Design review of the part built by this model. Coordinates are the model's own, in mm. A direction names the side the tool comes from. Give positions to 0.01 mm unless a question says otherwise; leave off trailing zeros. Order: outer loops, then holes, each group sorted by start corner. A loop starts at its lowest first (then second) coordinate and runs counter-clockwise, first axis right, second up. Notation, with made-up numbers: (24, 59) -> (30, 59) arc R21 ccw to (30, 76) -> close; hole circle Ø8 at (28, 74.5). An arc over 180 degrees is marked (long way). One line per item, written item: value. Start each with the question number.
1) Consider section C-C (z = -2.75). State how many separate pieces and enclosed holes the cut face has, plus the area to 3 significant figures.
2) Wall thickness on line 1 along Y through (x, z) = (30, 3.25); line 2 along Y through (x, z) = (70, -2.5); line 3 along Y through (x, z) = (11.5, 4.5): over which ranges is each line inside the solid? List them lowest first. Write a range as from..to.
3) Tool access review of faces 1 (the face through (20, 40, 2)), 2 (the face through (39, 41, -4.762)), 3 (the face through (57, 41, 0)), 4 (the face through (20, 20, -2)), 5 (the face through (40, 60, 2)): name each direction out of +Z, -Z, +X, -X, +Y, -Y from which nothing blocks a thin tool from reaching the whole face with its end or side.
4) For pin 1 (2 mm diameter, centred on y = 46.5, z = -1, fed in from -X); pin 2 (7 mm diameter, centred on x = 70, y = 30, fed in from +Z); pin 3 (4 mm diameter, centred on x = 18, z = 3.5, fed in from -Y), all flat-tipped, find the tip position at first contact; note any pin that passes through.
5) Consider section B-B (x = 30). State the section outline as (y, z) points.
6) Consider section A-A (y = 50). State the section outline as (x, z) points.
7) Consider section D-D (y = 30). State the section outline as (x, z) points.
8) The part is to be moulded in two halves that separate along X. For faces 6 (the face through (20, 60, 5)), 7 (the face through (67.973, 71.859, -2.415)), 8 (the face through (80, 39, -2)), say which applies: released by +X, released by -X, zero draft, split by the parting line, or undercut.
from build123d import *
from build123d.topology import SkipClean

# Parameters (mm, degrees)
SKETCH1_W                   = 40
SKETCH1_H                   = 40
BOSS_EXTRUDE1_DEPTH         = 4.7625
SKETCH1_3_W                 = 40
SKETCH1_3_H                 = 40
BOSS_EXTRUDE2_DEPTH         = 5
M5_CLEARANCE_HOLE1_D        = 5.5
BODY_MOVE_COPY1_OUTLINE_R   = 2.75
BODY_MOVE_COPY1_DEPTH       = 4.7625
BODY_MOVE_COPY1_START       = -5
BODY_MOVE_COPY1_2_OUTLINE_W = 40
BODY_MOVE_COPY1_2_OUTLINE_H = 40
BODY_MOVE_COPY1_2_OUTLINE_R = 2.75
BODY_MOVE_COPY1_2_DEPTH     = 0.2375
BODY_MOVE_COPY1_START_2     = -4.7625
BODY_MOVE_COPY1_3_OUTLINE_R = 2.75
BODY_MOVE_COPY1_3_DEPTH     = 4.7625
BODY_MOVE_COPY1_START_3     = 4.7625
BODY_MOVE_COPY1_4_OUTLINE_W = 40
BODY_MOVE_COPY1_4_OUTLINE_H = 40
BODY_MOVE_COPY1_4_OUTLINE_R = 2.75
BODY_MOVE_COPY1_4_DEPTH     = 0.2375


# Read off the part's stored shape, not the designer's step: Body-Move/Copy1
with BuildPart() as part:
    # Sketch1 → Boss-Extrude1 (new body)
    with BuildSketch(Plane.XY):
        with Locations((20, 60)):
            Rectangle(SKETCH1_W, SKETCH1_H)
        with Locations((60, 60)):
            Rectangle(SKETCH1_W, SKETCH1_H)
        with Locations((60, 20)):
            Rectangle(SKETCH1_W, SKETCH1_H)
        Polygon((40, 40), (0, 40), (40, 0), align=None)
    extrude(amount=BOSS_EXTRUDE1_DEPTH)

    # Sketch1<3> → Boss-Extrude2 (add)
    with BuildSketch(Plane.XY):
        with Locations((20, 60)):
            Rectangle(SKETCH1_3_W, SKETCH1_3_H)
    extrude(amount=-BOSS_EXTRUDE2_DEPTH)

    # M5 Clearance Hole1 (through all)
    with Locations(Plane.XY.offset(4.7625)):
        with Locations((10, 70), (30, 70), (50, 70), (70, 70), (30, 50), (50, 50), (70, 50), (30, 30), (50, 30), (70, 30), (50, 10), (70, 10), (10, 50)):
            Hole(M5_CLEARANCE_HOLE1_D / 2)

    # Body-Move/Copy1 outline → Body-Move/Copy1 (cut)
    with BuildSketch(Plane.XY):
        Polygon((40, 0), (80, 0), (80, 80), (40, 80), (40, 40), (0, 40), align=None)
        with Locations((30, 30)):
            Circle(BODY_MOVE_COPY1_OUTLINE_R, mode=Mode.SUBTRACT)
        with Locations((50, 10)):
            Circle(BODY_MOVE_COPY1_OUTLINE_R, mode=Mode.SUBTRACT)
        with Locations((70, 10)):
            Circle(BODY_MOVE_COPY1_OUTLINE_R, mode=Mode.SUBTRACT)
        with Locations((50, 30)):
            Circle(BODY_MOVE_COPY1_OUTLINE_R, mode=Mode.SUBTRACT)
        with Locations((70, 30)):
            Circle(BODY_MOVE_COPY1_OUTLINE_R, mode=Mode.SUBTRACT)
        with Locations((50, 50)):
            Circle(BODY_MOVE_COPY1_OUTLINE_R, mode=Mode.SUBTRACT)
        with Locations((70, 50)):
            Circle(BODY_MOVE_COPY1_OUTLINE_R, mode=Mode.SUBTRACT)
        with Locations((50, 70)):
            Circle(BODY_MOVE_COPY1_OUTLINE_R, mode=Mode.SUBTRACT)
        with Locations((70, 70)):
            Circle(BODY_MOVE_COPY1_OUTLINE_R, mode=Mode.SUBTRACT)
    extrude(amount=BODY_MOVE_COPY1_DEPTH, mode=Mode.SUBTRACT)

    # Body-Move_Copy1 2 outline → Body-Move_Copy1 2 (cut)
    with BuildSketch(Plane.XY.offset(BODY_MOVE_COPY1_START)):
        with Locations((20, 60)):
            Rectangle(BODY_MOVE_COPY1_2_OUTLINE_W, BODY_MOVE_COPY1_2_OUTLINE_H)
        with Locations((10, 50)):
            Circle(BODY_MOVE_COPY1_2_OUTLINE_R, mode=Mode.SUBTRACT)
        with Locations((30, 50)):
            Circle(BODY_MOVE_COPY1_2_OUTLINE_R, mode=Mode.SUBTRACT)
        with Locations((10, 70)):
            Circle(BODY_MOVE_COPY1_2_OUTLINE_R, mode=Mode.SUBTRACT)
        with Locations((30, 70)):
            Circle(BODY_MOVE_COPY1_2_OUTLINE_R, mode=Mode.SUBTRACT)
    extrude(amount=BODY_MOVE_COPY1_2_DEPTH, mode=Mode.SUBTRACT)

    # Body-Move_Copy1 3 outline → Body-Move_Copy1 3 (add)
    with BuildSketch(Plane.XY.offset(BODY_MOVE_COPY1_START_2)):
        Polygon((40, 0), (80, 0), (80, 80), (40, 80), (40, 40), (0, 40), align=None)
        with Locations((30, 30)):
            Circle(BODY_MOVE_COPY1_3_OUTLINE_R, mode=Mode.SUBTRACT)
        with Locations((50, 10)):
            Circle(BODY_MOVE_COPY1_3_OUTLINE_R, mode=Mode.SUBTRACT)
        with Locations((70, 10)):
            Circle(BODY_MOVE_COPY1_3_OUTLINE_R, mode=Mode.SUBTRACT)
        with Locations((50, 30)):
            Circle(BODY_MOVE_COPY1_3_OUTLINE_R, mode=Mode.SUBTRACT)
        with Locations((70, 30)):
            Circle(BODY_MOVE_COPY1_3_OUTLINE_R, mode=Mode.SUBTRACT)
        with Locations((50, 50)):
            Circle(BODY_MOVE_COPY1_3_OUTLINE_R, mode=Mode.SUBTRACT)
        with Locations((70, 50)):
            Circle(BODY_MOVE_COPY1_3_OUTLINE_R, mode=Mode.SUBTRACT)
        with Locations((50, 70)):
            Circle(BODY_MOVE_COPY1_3_OUTLINE_R, mode=Mode.SUBTRACT)
        with Locations((70, 70)):
            Circle(BODY_MOVE_COPY1_3_OUTLINE_R, mode=Mode.SUBTRACT)
    extrude(amount=BODY_MOVE_COPY1_3_DEPTH)

    # Body-Move_Copy1 4 outline → Body-Move_Copy1 4 (add)
    with SkipClean():  # the faces are left unmerged after this step: merging them gives an invalid solid
        with BuildSketch(Plane.XY.offset(BODY_MOVE_COPY1_START_3)):
            with Locations((20, 60)):
                Rectangle(BODY_MOVE_COPY1_4_OUTLINE_W, BODY_MOVE_COPY1_4_OUTLINE_H)
            with Locations((10, 50)):
                Circle(BODY_MOVE_COPY1_4_OUTLINE_R, mode=Mode.SUBTRACT)
            with Locations((30, 50)):
                Circle(BODY_MOVE_COPY1_4_OUTLINE_R, mode=Mode.SUBTRACT)
            with Locations((10, 70)):
                Circle(BODY_MOVE_COPY1_4_OUTLINE_R, mode=Mode.SUBTRACT)
            with Locations((30, 70)):
                Circle(BODY_MOVE_COPY1_4_OUTLINE_R, mode=Mode.SUBTRACT)
        extrude(amount=BODY_MOVE_COPY1_4_DEPTH)
    add(part.part.scale(1), mode=Mode.REPLACE)  # the faces are merged on a copy


solid = part.part
Checked values:
1. separate pieces: 1
1. enclosed holes: 13
1. area: 5,290 mm^2
2. line 1: y = 40..47.25, 52.75..67.25, 72.75..80
2. line 2: y = 0..7.25, 12.75..27.25, 32.75..47.25, 52.75..67.25, 72.75..80
2. line 3: y = 40..47.7, 52.3..67.7, 72.3..80
3. face 1: +Z, +X, -X, -Y
3. face 2: -Z, +X, -X, +Y, -Y
3. face 3: +Z, +X, -Y
3. face 4: +Z, -Z, -X, -Y
3. face 5: +Z, +X, +Y, -Y
4. pin 1: stops at x = 0
4. pin 2: stops at z = 0
4. pin 3: stops at y = 40
5. outline: (10, -4.76) -> (27.25, -4.76) -> (27.25, 0) -> (10, 0) -> close; (32.75, -4.76) -> (47.25, -4.76) -> (47.25, 5) -> (40, 5) -> (40, 0) -> (32.75, 0) -> close; (52.75, -4.76) -> (67.25, -4.76) -> (67.25, 5) -> (52.75, 5) -> close; (72.75, -4.76) -> (80, -4.76) -> (80, 5) -> (72.75, 5) -> close
6. outline: (0, -4.76) -> (7.25, -4.76) -> (7.25, 5) -> (0, 5) -> close; (12.75, -4.76) -> (27.25, -4.76) -> (27.25, 5) -> (12.75, 5) -> close; (32.75, -4.76) -> (47.25, -4.76) -> (47.25, 0) -> (40, 0) -> (40, 5) -> (32.75, 5) -> close; (52.75, -4.76) -> (67.25, -4.76) -> (67.25, 0) -> (52.75, 0) -> close; (72.75, -4.76) -> (80, -4.76) -> (80, 0) -> (72.75, 0) -> close
7. outline: (10, -4.76) -> (27.25, -4.76) -> (27.25, 0) -> (10, 0) -> close; (32.75, -4.76) -> (47.25, -4.76) -> (47.25, 0) -> (32.75, 0) -> close; (52.75, -4.76) -> (67.25, -4.76) -> (67.25, 0) -> (52.75, 0) -> close; (72.75, -4.76) -> (80, -4.76) -> (80, 0) -> (72.75, 0) -> close
8. face 6: zero draft
8. face 7: undercut
8. face 8: released by +X
